from build123d import *

# Parameters (mm, degrees)
SKETCH2_R           = 1.65
SKETCH2_R_2         = 1.929414359
BOSS_EXTRUDE1_DEPTH = 3


with BuildPart() as part:
    # Sketch2 → Boss-Extrude1 (new body)
    with BuildSketch(Plane.XY):
        Polygon((32.568394145, 0), (-33.272239932, -0.000293688), (-27.618837956, -30), (-13.191429734, -49.85768247), (12.487583947, -49.85768247), (26.91499217, -30), align=None)
        with Locations((-9.342728507, -42.860194395)):
            Circle(SKETCH2_R, mode=Mode.SUBTRACT)
        with Locations((8.490760277, -42.860194395)):
            Circle(SKETCH2_R, mode=Mode.SUBTRACT)
        with Locations((-12.933964176, -10.050384435)):
            Circle(SKETCH2_R, mode=Mode.SUBTRACT)
        with Locations((12.487583947, -9.80768247)):
            Circle(SKETCH2_R_2, mode=Mode.SUBTRACT)
    extrude(amount=BOSS_EXTRUDE1_DEPTH)


solid = part.part
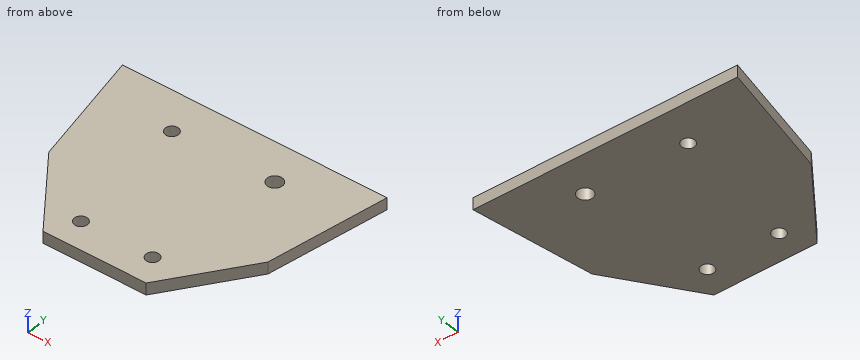
Geometry: final body of the model. Coordinates: model frame, mm. Give positions to 0.01 mm unless a question says otherwise; leave off trailing zeros. Write each loop counter-clockwise with the first axis right and the second up, starting at its lowest first coordinate (ties: lowest second). Pieces come first, ordered by that corner, then holes. Notation, with made-up numbers: (49.25, 60) -> (71.25, 60) arc R16 cw to (71.25, 77) -> close; hole circle Ø5 at (47, 78.25). An arc over 180 degrees is marked (long way). Answer in a Markdown table with one row per item.
(1) Section query D-D on y = -6. Return loops of the section in (x, z).
Answers below:
| item | result |
|---|---|
| outline | (-32.14, 0) -> (31.44, 0) -> (31.44, 3) -> (-32.14, 3) -> close |
(2) Section query B-B on z = 1.9. Return loops of the section in (x, y) (3 decimals).
Answers below:
| item | result |
|---|---|
| outline | (-33.272, 0) -> (-27.619, -30) -> (-13.191, -49.858) -> (12.488, -49.858) -> (26.915, -30) -> (32.568, 0) -> close; hole circle Ø3.3 at (-12.934, -10.05); hole circle Ø3.3 at (-9.343, -42.86); hole circle Ø3.3 at (8.491, -42.86); hole circle Ø3.859 at (12.488, -9.808) |
(3) Ray query, line 1 along X through (y, z) = (-43, 0.3); line 2 along X through (y, z) = (-11.5, 2.45); line 3 along X through (y, z) = (-17, 1.45). Return the intervals inside material, ascending. Write a range as [from, to].
Answers below:
| item | result |
|---|---|
| line 1 | [-18.17, -10.99], [-7.7, 6.85], [10.13, 17.47] |
| line 2 | [-31.11, -13.72], [-12.15, 11.56], [13.41, 30.4] |
| line 3 | [-30.07, 29.36] |
(4) Section query A-A on y = -11. Return loops of the section in (x, z).
Answers below:
| item | result |
|---|---|
| outline | (-31.2, 0) -> (-14.28, 0) -> (-14.28, 3) -> (-31.2, 3) -> close; (-11.58, 0) -> (10.97, 0) -> (10.97, 3) -> (-11.58, 3) -> close; (14, 0) -> (30.5, 0) -> (30.5, 3) -> (14, 3) -> close |
(5) Section query C-C on x = -26.5. Return loops of the section in (y, z).
Answers below:
| item | result |
|---|---|
| outline | (-31.54, 0) -> (0, 0) -> (0, 3) -> (-31.54, 3) -> close |
